```python
from build123d import *

# Parameters (mm, degrees)
SKETCH1_W           = 272
SKETCH1_H           = 56
BOSS_EXTRUDE1_DEPTH = 3
CUT_EXTRUDE1_REACH  = 275.454
SKETCH4_R           = 1.6
SKETCH4_W           = 20
SKETCH4_H           = 20
SKETCH5_W           = 3
SKETCH5_H           = 30
SKETCH5_W_2         = 30
SKETCH5_H_2         = 3
BOSS_EXTRUDE2_DEPTH = 3


with BuildPart() as part:
    # Sketch1 → Boss-Extrude1 (new body)
    with BuildSketch(Plane.XY):
        with Locations((136, 0)):
            Rectangle(SKETCH1_W, SKETCH1_H)
    extrude(amount=BOSS_EXTRUDE1_DEPTH)

    # Sketch4 → Cut-Extrude1 (cut, up to next)
    with BuildSketch(Plane.XY.offset(3), mode=Mode.PRIVATE) as cut_extrude1_sk1:
        with Locations((253.41, -10.06)):
            Circle(SKETCH4_R)
    cut_extrude1_tool1 = extrude(cut_extrude1_sk1.sketch, amount=-CUT_EXTRUDE1_REACH, mode=Mode.PRIVATE) & part.part
    # Sketch4 → Cut-Extrude1 (cut, up to next)
    with BuildSketch(Plane.XY.offset(3), mode=Mode.PRIVATE) as cut_extrude1_sk2:
        with Locations((253.41, 4.02)):
            Circle(SKETCH4_R)
    cut_extrude1_tool2 = extrude(cut_extrude1_sk2.sketch, amount=-CUT_EXTRUDE1_REACH, mode=Mode.PRIVATE) & part.part
    # Sketch4 → Cut-Extrude1 (cut, up to next)
    with BuildSketch(Plane.XY.offset(3), mode=Mode.PRIVATE) as cut_extrude1_sk3:
        with Locations((113, -10.06)):
            Circle(SKETCH4_R)
    cut_extrude1_tool3 = extrude(cut_extrude1_sk3.sketch, amount=-CUT_EXTRUDE1_REACH, mode=Mode.PRIVATE) & part.part
    # Sketch4 → Cut-Extrude1 (cut, up to next)
    with BuildSketch(Plane.XY.offset(3), mode=Mode.PRIVATE) as cut_extrude1_sk4:
        with Locations((10, -18)):
            Rectangle(SKETCH4_W, SKETCH4_H)
    cut_extrude1_tool4 = extrude(cut_extrude1_sk4.sketch, amount=-CUT_EXTRUDE1_REACH, mode=Mode.PRIVATE) & part.part
    add(cut_extrude1_tool1.solids().sort_by_distance((253.41, -10.06, 3))[0], mode=Mode.SUBTRACT)
    add(cut_extrude1_tool2.solids().sort_by_distance((253.41, 4.02, 3))[0], mode=Mode.SUBTRACT)
    add(cut_extrude1_tool3.solids().sort_by_distance((113, -10.06, 3))[0], mode=Mode.SUBTRACT)
    add(cut_extrude1_tool4.solids().sort_by_distance((10, -18, 3))[0], mode=Mode.SUBTRACT)

    # Sketch5 → Boss-Extrude2 (add)
    with BuildSketch(Plane.XY):
        with Locations((273.5, 0)):
            Rectangle(SKETCH5_W, SKETCH5_H)
        with Locations((212, 29.5)):
            Rectangle(SKETCH5_W_2, SKETCH5_H_2)
        with Locations((152, 29.5)):
            Rectangle(SKETCH5_W_2, SKETCH5_H_2)
        with Locations((92, 29.5)):
            Rectangle(SKETCH5_W_2, SKETCH5_H_2)
        with Locations((32, 29.5)):
            Rectangle(SKETCH5_W_2, SKETCH5_H_2)
        with Locations((242, -29.5)):
            Rectangle(SKETCH5_W_2, SKETCH5_H_2)
        with Locations((182, -29.5)):
            Rectangle(SKETCH5_W_2, SKETCH5_H_2)
        with Locations((122, -29.5)):
            Rectangle(SKETCH5_W_2, SKETCH5_H_2)
        with Locations((62, -29.5)):
            Rectangle(SKETCH5_W_2, SKETCH5_H_2)
    extrude(amount=BOSS_EXTRUDE2_DEPTH)

    # Mirror1: part across plane


with BuildPart() as part_1:
    add(part.part)
    add(part.part.mirror(Plane(origin=(0, -28, 3), x_dir=(0, 0, 1), z_dir=(1, 0, 0))))


solid = part_1.part
```
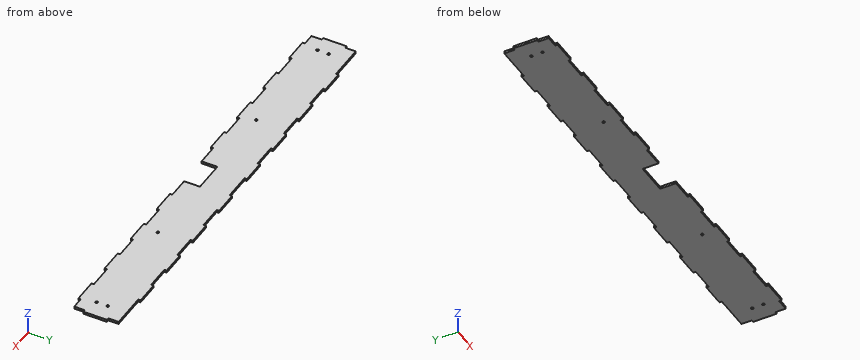
Can you work these out from the model? Positions are in its coordinate system, mm. Give positions to 0.01 mm unless a question says otherwise; leave off trailing zeros. Loops run counter-clockwise (first coordinate to the right, second up) from the corner with the lowest first, then second, coordinate; pieces in that order, holes last. Notation, with made-up numbers: M 13,4 L 31,4 A35 ccw 31,37 Z; hole C 33,61 d7. An arc over 180 degrees is marked long. One line per item, written item: value.
(1) Suppose I cut it at A-A on z = 1.6. Count the separate pieces of the cut face and the enclosed holes in it, plus the area to 3 significant figures.
Returned:
separate pieces: 1
enclosed holes: 6
area: 31,200 mm^2
(2) Will these pins go through, and if not, where does the flat tip stop? pin 1 (1.5 mm diameter, centred on y = -29, z = 2, fed in from +X); pin 2 (1.5 mm diameter, centred on y = 29, z = 2, fed in from -X); pin 3 (1.9 mm diameter, centred on x = -113, y = -10.06, fed in from -Z); pin 4 (1 mm diameter, centred on x = 149.5, z = 0.5, fed in from -Y).
Returned:
pin 1: x = 257
pin 2: x = -227
pin 3: through
pin 4: y = -28
(3) Suppose I cut it at B-B on x = 219. List the corners of the cut face in (y, z) for me, plus the area to 3 significant figures.
Returned:
outline: M -28,0 L 31,0 L 31,3 L -28,3 Z
area: 177 mm^2
(4) I need wall thicknesses on line 1 (Y direction, x = -253.41, z = 2.35); line 2 (X direction, y = -22, z = 0.9); line 3 (Y direction, x = 113, z = 1.95). Which ranges of each line are inside material? Lowest first, please.
Returned:
line 1: -31 to -11.66, -8.46 to 2.42, 5.62 to 28
line 2: -272 to -20, 20 to 272
line 3: -31 to -11.66, -8.46 to 28
